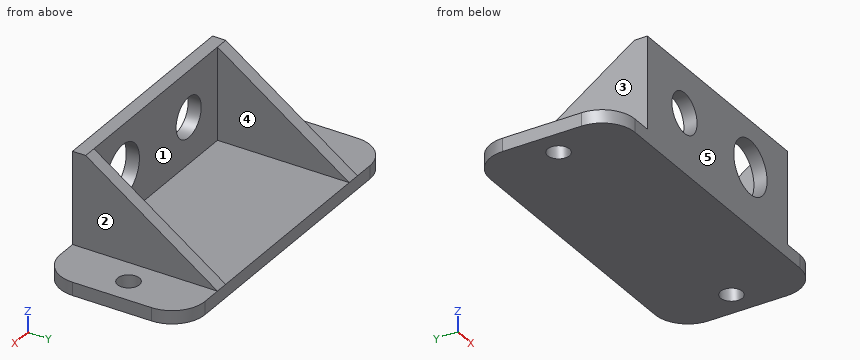
```python
from build123d import *

# Parameters (mm, degrees)
F0_W      = 50
F0_H      = 22
F1_DEPTH  = 2
F2_W      = 34
F2_H      = 2
F3_DEPTH  = 14
F4_R      = 3.05
F4_R_2    = 4.05
F5_DEPTH  = 2
F6_R      = 1.65
F7_DEPTH  = 2
F9_DEPTH  = 2
F11_DEPTH = 2
F12_R     = 5
F13_R     = 5


with BuildPart() as f1:
    # F0 (on Top) → F1 (new body)
    with BuildSketch(Plane.XY):
        Rectangle(F0_W, F0_H)
    extrude(amount=F1_DEPTH)

    # F2 (on face) → F3 (join)
    with BuildSketch(Plane.XY.offset(2)):
        with Locations((0, -10)):
            Rectangle(F2_W, F2_H)
    extrude(amount=F3_DEPTH)

    # F4 (on face) → F5 (cut)
    with BuildSketch(Plane.XZ.offset(11)):
        with Locations((-8, 9)):
            Circle(F4_R)
        with Locations((8, 9)):
            Circle(F4_R_2)
    extrude(amount=-F5_DEPTH, mode=Mode.SUBTRACT)

    # F6 (on face) → F7 (cut)
    with BuildSketch(Plane.XY.offset(2)):
        with Locations((-21, 0)):
            Circle(F6_R)
        with Locations((21, 0)):
            Circle(F6_R)
    extrude(amount=-F7_DEPTH, mode=Mode.SUBTRACT)

    # F8 (on face) → F9 (join)
    with BuildSketch(Plane.YZ.offset(17)):
        Polygon((10.999476, 1.999592), (-9, 16), (-9, 2), align=None)
    extrude(amount=-F9_DEPTH)

    # F10 (on face) → F11 (join)
    with BuildSketch(Plane(origin=(-17, 0, 0), x_dir=(0, -1, 0), z_dir=(-1, 0, 0))):
        Polygon((9, 2), (9, 16), (-10.999475, 1.999864), align=None)
    extrude(amount=-F11_DEPTH)

    # F12
    f12_edges = [f1.edges().sort_by_distance(p)[0] for p in [
        (-25, 11, 1),
        (-25, -11, 1),
    ]]
    fillet(f12_edges, radius=F12_R)

    # F13
    f13_edges = [f1.edges().sort_by_distance(p)[0] for p in [
        (25, -11, 1),
        (25, 11, 1),
    ]]
    fillet(f13_edges, radius=F13_R)


solid = f1.part
```
Part model, mm, in its own coordinate system. Face numbers are marked on the shaded views. A direction names the side the tool comes from. Round coordinates to 2 decimals unless told otherwise and drop trailing zeros. Loops run counter-clockwise (first coordinate to the right, second up) from the corner with the lowest first, then second, coordinate; pieces in that order, holes last. Notation, with made-up numbers: (66.5, 36.25) -> (124.5, 36.25) arc R27 ccw to (124.5, 65.25) -> close; hole circle Ø1 at (63.25, 66.5). An arc over 180 degrees is marked (long way). Use CSV: the item, a comma, the result in double quotes. Start each with the question number.
1) Drop flat-ended pins along their axis: P1, Ø5, axis at y = 5.5, z = 5, coming from the -X side; P2, Ø5, axis at y = 1.5, z = 9, coming from the +X side; P3, Ø1.5, axis at y = -1, z = 13, coming from the +X side; P4, Ø4.5, axis at x = 21, y = 0, coming from the +Z side. Give the stop position or say it passes through.
2) Cut at C-C, the plane z = 11. Write the cut outline in (x, y), plus the area to 3 significant figures.
3) Cut at D-D, the plane y = 7.5. Write the cut outline in (x, z), plus the area to 3 significant figures.
4) Cut at B-B, the plane y = 0. Write the cut outline in (x, z), plus the area to 3 significant figures.
5) Cut at A-A, the plane x = -8. Write the cut outline in (y, z).
6) Wall check: L1, parallel to X at y = -7, z = 13; L2, parallel to Z at x = -8, y = -10.45; L3, parallel to Z at x = 8, y = -9.45. Give the ranges that are in metal, low to high. Write a range as [from, to].
7) Which spindle directions (+Z, -Z, +X, -X, +Y, -Y) get a long thin tool onto all of the face, cutting with end or side? Do the marked faces 4 and 5. Say none if no direction does.
8) Pull direction X, two halves, no side cores. Call the marked faces 1, 2 and 3: +X half, -X half, draft (parallel to the pull), parting line (faces both ways), or undercut.
Determined:
1,P1,"stops at x = -17"
1,P2,"stops at x = 17"
1,P3,"passes through"
1,P4,"stops at z = 2"
2,outline,"(-17, -11) -> (-10.3, -11) -> (-10.3, -9) -> (-15, -9) -> (-15, -1.86) -> (-17, -1.86) -> close; (-5.7, -11) -> (4.48, -11) -> (4.48, -9) -> (-5.7, -9) -> close; (11.52, -11) -> (17, -11) -> (17, -1.86) -> (15, -1.86) -> (15, -9) -> (11.52, -9) -> close"
2,area,"73.3 mm2"
3,outline,"(-24.77, 0) -> (24.77, 0) -> (24.77, 2) -> (17, 2) -> (17, 4.45) -> (15, 4.45) -> (15, 2) -> (-15, 2) -> (-15, 4.45) -> (-17, 4.45) -> (-17, 2) -> (-24.77, 2) -> close"
3,area,"109 mm2"
4,outline,"(-25, 0) -> (-22.65, 0) -> (-22.65, 2) -> (-25, 2) -> close; (-19.35, 0) -> (19.35, 0) -> (19.35, 2) -> (17, 2) -> (17, 9.7) -> (15, 9.7) -> (15, 2) -> (-15, 2) -> (-15, 9.7) -> (-17, 9.7) -> (-17, 2) -> (-19.35, 2) -> close; (22.65, 0) -> (25, 0) -> (25, 2) -> (22.65, 2) -> close"
4,area,"118 mm2"
5,outline,"(-11, 0) -> (11, 0) -> (11, 2) -> (-9, 2) -> (-9, 5.95) -> (-11, 5.95) -> close; (-11, 12.05) -> (-9, 12.05) -> (-9, 16) -> (-11, 16) -> close"
6,L1,"x = [-17, -15], [15, 17]"
6,L2,"z = [0, 5.95], [12.05, 16]"
6,L3,"z = [0, 4.95], [13.05, 16]"
7,face 4,"+Z, +Y"
7,face 5,"+Z, -Z, +X, -X, -Y"
8,face 1,"undercut"
8,face 2,"+X half"
8,face 3,"-X half"
